Source: three-view drawing plus pictorial views. Frame: mm from the lowest corner of the part. A direction names the side the tool comes from. Give positions to 0.01 mm unless a question says otherwise; leave off trailing zeros. Order: outer loops, then holes, each group sorted by start corner. A loop starts at its lowest first (then second) coordinate and runs counter-clockwise, first axis right, second up.
1) Section D-D, the plane x = 31. Return loops of the section in (y, z), plus the area to 3 significant figures.
2) Section B-B, the plane y = 25. Return loops of the section in (x, z), plus the area to 3 significant figures.
3) Section A-A, the plane x = 37.5. Return loops of the section in (y, z), plus the area to 3 significant figures.
4) Access query for the marked faces 4 and 5. Directions: +Z, -Z, +X, -X, +Y, -Y. A direction counts if a zero-diameter tool reaches every point of the face in a straight line with its end or side. Return the directions, or none.
5) Material intervals for line 1 (X direction, y = 2.65, z = 25); line 2 (X direction, y = 27, z = 4); line 3 (Y direction, x = 12.5, z = 3.85), sorted ascending.
6) Draft query along Z for the marked faces 1, 2 and 3. Return one class per face: released by +Z, released by -Z, zero draft, split by the parting line, or undercut.
7) First-contact query: P1, Ø8, axis at x = 37.5, y = 25, coming from the +Z side; P2, Ø7, axis at x = 37.5, z = 25, coming from the +Y side. Flat tips, straight axial feed; report the tip coordinate or a pass-through.
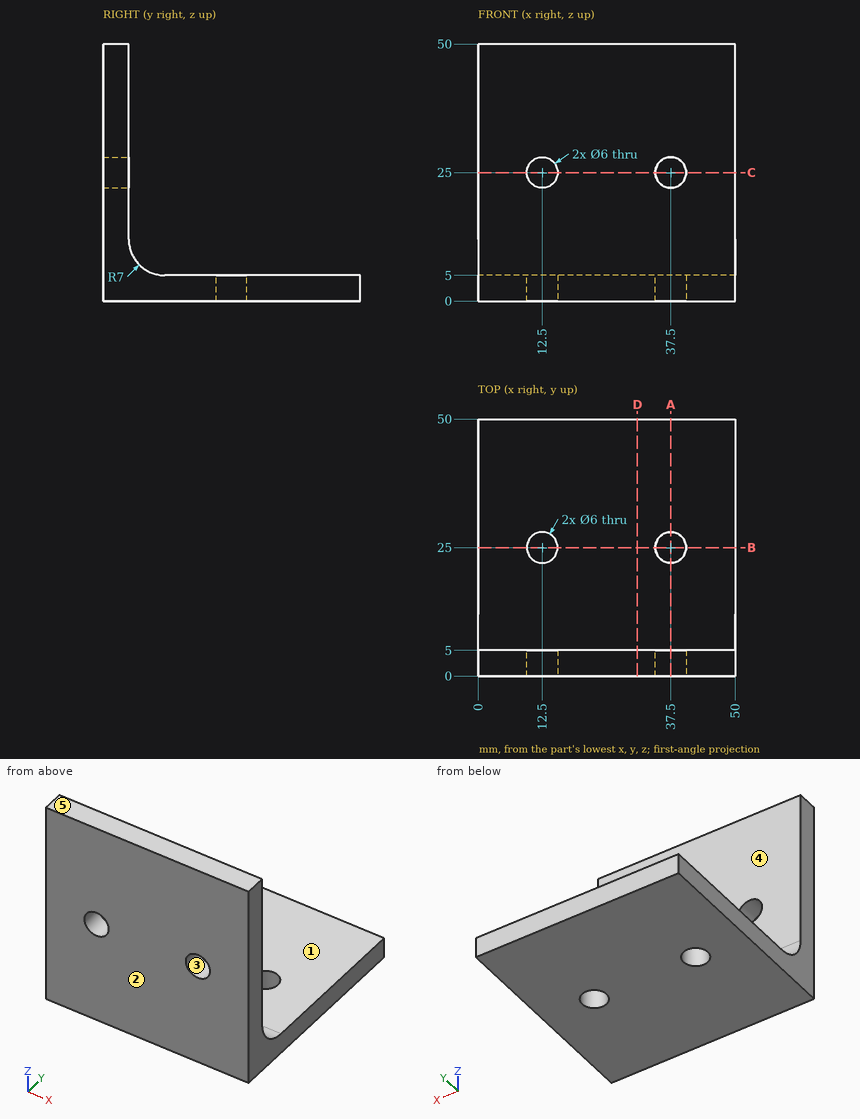
From the geometry:
1. outline: (0, 0) - (50, 0) - (50, 5) - (12, 5) arc R7 cw to (5, 12) - (5, 50) - (0, 50) - close
1. area: 486 mm2
2. outline: (0, 0) - (9.5, 0) - (9.5, 5) - (0, 5) - close; (15.5, 0) - (34.5, 0) - (34.5, 5) - (15.5, 5) - close; (40.5, 0) - (50, 0) - (50, 5) - (40.5, 5) - close
2. area: 190 mm2
3. outline: (0, 0) - (22, 0) - (22, 5) - (12, 5) arc R7 cw to (5, 12) - (5, 22) - (0, 22) - close; (0, 28) - (5, 28) - (5, 50) - (0, 50) - close; (28, 0) - (50, 0) - (50, 5) - (28, 5) - close
3. area: 426 mm2
4. face 4: +Z, +X, -X, +Y
4. face 5: +Z, +X, -X, +Y, -Y
5. line 1: x = 0 to 9.5, 15.5 to 34.5, 40.5 to 50
5. line 2: x = 0 to 10.26, 14.74 to 35.26, 39.74 to 50
5. line 3: y = 0 to 22, 28 to 50
6. face 1: released by +Z
6. face 2: zero draft
6. face 3: undercut
7. P1: stops at z = 5
7. P2: stops at y = 5
